```python
from build123d import *

# Parameters (mm, degrees)
F0_W     = 24.3
F0_H     = 10.7
F0_W_2   = 20.3
F0_H_2   = 6.7
F1_DEPTH = 11.15
F2_W     = 20.3
F2_H     = 6.7
F2_W_2   = 18.3
F2_H_2   = 4.7
F3_DEPTH = 1
F5_DEPTH = 20


with BuildPart() as f1:
    # F0 (on Front) → F1 (new body)
    with BuildSketch(Plane.XZ):
        Rectangle(F0_W, F0_H)
        Rectangle(F0_W_2, F0_H_2, mode=Mode.SUBTRACT)
    extrude(amount=F1_DEPTH)

    # F2 (on face) → F3 (join)
    with BuildSketch(Plane.XZ.offset(11.15)):
        Rectangle(F2_W, F2_H)
        Rectangle(F2_W_2, F2_H_2, mode=Mode.SUBTRACT)
    extrude(amount=-F3_DEPTH)

    # F4 (on face) → F5 (join)
    with BuildSketch(Plane.XZ.offset(11.15)):
        Polygon((12.15, 2.35), (12.15, 5.35), (-12.15, 5.35), (-12.15, 2.35), (-9.15, 2.35), (9.15, 2.35), align=None)
    extrude(amount=F5_DEPTH)


solid = f1.part
```
Source: CAD feature listing. Evaluate the final solid. Frame: model axes, mm. A direction names the side the tool comes from. Give positions to 0.01 mm unless a question says otherwise; leave off trailing zeros. Write each loop counter-clockwise with the first axis right and the second up, starting at its lowest first coordinate (ties: lowest second). Pieces come first, ordered by that corner, then holes. Notation, with made-up numbers: (29.25, 37.5) - (75.25, 37.5) arc R27 ccw to (75.25, 64.5) - close; hole circle Ø5 at (48.5, 43). An arc over 180 degrees is marked (long way). One line per item, written item: value. Start each with the question number.
Q1. First-contact query: pin 1 Ø4 at (x, z) = (-3, -2) entering from -Y; pin 2 Ø6.5 at (x, y) = (4, -20) entering from -Z. Flat tips, straight axial feed; report the tip coordinate or a pass-through.
Q2. Section query B-B, the plane x = -1.5. Return the cut outline in (y, z), then the cut area to 3 significant figures.
Q3. Draft query along X for faces 1 (the face through (0, 0, 4)), 2 (the face through (0, -11, -2.35)), 3 (the face through (-12.15, -12, 4)). Return one class per face: +X half, -X half, draft (parallel to the pull), parting line (faces both ways), or undercut.
Q4. Section query A-A, the plane z = 0. Return the cut outline in (x, y).
Q5. Section query C-C, the plane y = -4.5. Return the cut outline in (x, z).
Q6. Set-up query: faces 4 (the face through (-9.15, -11, 0)), 5 (the face through (0, -5, -3.35)), 6 (the face through (0, -15, 5.35)), 7 (the face through (0, -11.15, -3)), 8 (the face through (12.15, -8, 1)). Return all of +Z, -Z, +X, -X, +Y, -Y with unobstructed straight access to the full face (end or side cutting, diameter ignored); none if empty.
Q7. Material intervals for probe 1 along Z at (x, y) = (-9, -10.5); probe 2 along Z at (x, y) = (10, -2); probe 3 along X at (y, z) = (-2, 2), sorted ascending. Write a range as from..to.
Q8. Section query D-D, the plane z = 3. Return the cut outline in (x, y), then the cut area to 3 significant figures.
Answer:
1. pin 1: stops at y = -11.15
1. pin 2: stops at z = 2.35
2. outline: (-31.15, 2.35) - (-10.15, 2.35) - (-10.15, 3.35) - (0, 3.35) - (0, 5.35) - (-31.15, 5.35) - close; (-11.15, -5.35) - (0, -5.35) - (0, -3.35) - (-10.15, -3.35) - (-10.15, -2.35) - (-11.15, -2.35) - close
2. area: 107 mm2
3. face 1: draft
3. face 2: undercut
3. face 3: -X half
4. outline: (-12.15, -11.15) - (-9.15, -11.15) - (-9.15, -10.15) - (-10.15, -10.15) - (-10.15, 0) - (-12.15, 0) - close; (9.15, -11.15) - (12.15, -11.15) - (12.15, 0) - (10.15, 0) - (10.15, -10.15) - (9.15, -10.15) - close
5. outline: (-12.15, -5.35) - (12.15, -5.35) - (12.15, 5.35) - (-12.15, 5.35) - close; hole (-10.15, -3.35) - (10.15, -3.35) - (10.15, 3.35) - (-10.15, 3.35) - close
6. face 4: +Y, -Y
6. face 5: +Y
6. face 6: +Z, +X, -X, +Y, -Y
6. face 7: -Z, +X, -X, -Y
6. face 8: +Z, -Z, +X, +Y, -Y
7. probe 1: z = -5.35..-2.35, 2.35..5.35
7. probe 2: z = -5.35..-3.35, 3.35..5.35
7. probe 3: x = -12.15..-10.15, 10.15..12.15
8. outline: (-12.15, -31.15) - (12.15, -31.15) - (12.15, 0) - (10.15, 0) - (10.15, -10.15) - (-10.15, -10.15) - (-10.15, 0) - (-12.15, 0) - close
8. area: 551 mm2
